Check sheet for the drawn part. Datum: minimum x, y, z corner. Units: mm. A direction names the side the tool comes from. Round coordinates to 2 decimals unless told otherwise and drop trailing zeros. Write each loop counter-clockwise with the first axis right and the second up, starting at its lowest first coordinate (ties: lowest second). Pieces come first, ordered by that corner, then holes. Notation, with made-up numbers: M -33,-2 L 13,-2 A14 ccw 13,15 Z; hole C 54.25,49 d6. An arc over 180 degrees is marked long. One line per item, written item: value. Start each with the question number.
Item 1: Section check B-B, the plane x = 10. Record the cut outline in (y, z).
Item 2: Thickness scan on probe 1 along X at (y, z) = (5.5, 6); probe 2 along Y at (x, z) = (16.5, 10.75); probe 3 along Z at (x, y) = (9, 12.25). Record the ranges inside material, lowest first. Write a range as from..to.
Item 3: Section check D-D, the plane z = 4.5. Record the cut outline in (x, y).
Item 4: Section check A-A, the plane z = 15. Record the cut outline in (x, y).
Item 5: Tool access check on the marked faces 1, 2 and 3. Record the directions out of +Z, -Z, +X, -X, +Y, -Y that give a thin tool (end or side, any length) a straight path to the whole face; none if there is none.
Item 6: Gauge pin test, flat ends, axial feed: pin 1 (1.6 mm diameter, centred on x = 18.5, z = 13, fed in from -Y); pin 2 (4 mm diameter, centred on y = 3.5, z = 9, fed in from +X); pin 3 (2 mm diameter, centred on x = 19, z = 12.5, fed in from +Y); pin 4 (1 mm diameter, centred on x = 15, y = 10.5, fed in from +Z). Record the tip position at first contact, or that the pin passes through.
Item 7: Section check C-C, the plane y = 11.75. Record the cut outline in (x, z), then the cut area to 3 significant figures.
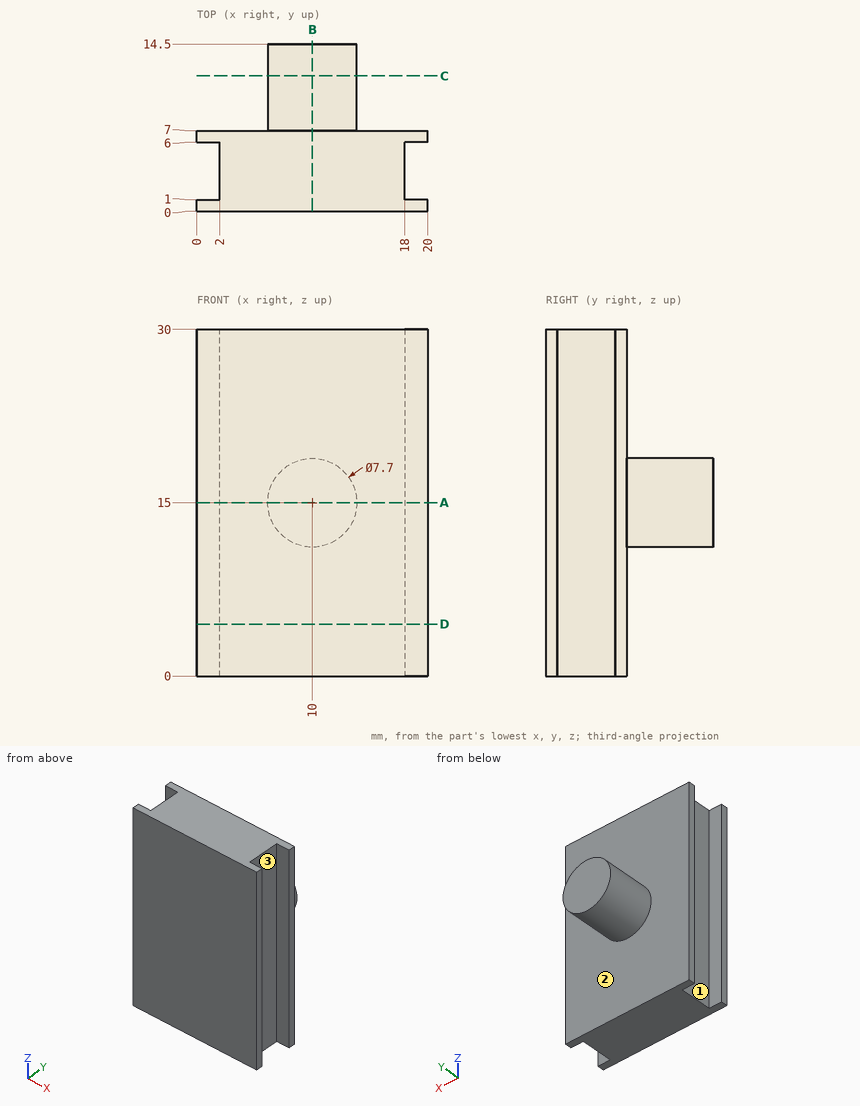
Response values:
1. outline: M 0,0 L 7,0 L 7,11.15 L 14.5,11.15 L 14.5,18.85 L 7,18.85 L 7,30 L 0,30 Z
2. probe 1: x = 2..18
2. probe 2: y = 0..7
2. probe 3: z = 11.28..18.72
3. outline: M 0,0 L 20,0 L 20,1 L 18,1 L 18,6 L 20,6 L 20,7 L 0,7 L 0,6 L 2,6 L 2,1 L 0,1 Z
4. outline: M 0,0 L 20,0 L 20,1 L 18,1 L 18,6 L 20,6 L 20,7 L 13.85,7 L 13.85,14.5 L 6.15,14.5 L 6.15,7 L 0,7 L 0,6 L 2,6 L 2,1 L 0,1 Z
5. face 1: +Z, -Z, -X
5. face 2: +Y
5. face 3: +Z, -Z, +X
6. pin 1: stops at y = 0
6. pin 2: stops at x = 18
6. pin 3: stops at y = 7
6. pin 4: passes through
7. outline: C 10,15 d7.7
7. area: 46.6 mm2
